Can you work these out from the model? Positions are in its coordinate system, mm. A direction names the side the tool comes from. Give positions to 0.01 mm unless a question says otherwise; leave off trailing zeros. Order: outer loops, then holes, each group sorted by start corner. A loop starts at its lowest first (then second) coordinate and runs counter-clockwise, first axis right, second up. Notation, with made-up numbers: (38.5, 64.25) - (84.5, 64.25) arc R18 ccw to (84.5, 90.25) - close; hole circle Ø2 at (0.5, 20). An arc over 180 degrees is marked (long way). Answer as CSV lines item,"result".
```python
from build123d import *

# Parameters (mm, degrees)
SKETCH1_W           = 24.825
SKETCH1_H           = 3.175
SKETCH1_W_2         = 3.175
SKETCH1_H_2         = 24.825
BOSS_EXTRUDE1_DEPTH = 60
SKETCH2_W           = 3.125
SKETCH2_H           = 5.4
BOSS_EXTRUDE4_DEPTH = 3.175
SKETCH4_R           = 8
CUT_EXTRUDE1_DEPTH  = 3.175
SKETCH3_R           = 8
CUT_EXTRUDE2_DEPTH  = 3.175
SKETCH5_W           = 3.175
SKETCH5_H           = 5.4
BOSS_EXTRUDE5_DEPTH = 3.175
SKETCH6_R           = 1.75
CUT_EXTRUDE3_DEPTH  = 10
SKETCH7_R           = 1.75
CUT_EXTRUDE4_DEPTH  = 10


with BuildPart() as part:
    # Sketch1 → Boss-Extrude1 (new body)
    with BuildSketch(Plane(origin=(0, 0, 0), x_dir=(1, 0, 0), z_dir=(0, 1, 0))):
        with Locations((-38.0875, 24.0875)):
            Rectangle(SKETCH1_W, SKETCH1_H)
        with Locations((-24.0875, 24.0875)):
            Rectangle(SKETCH1_W_2, SKETCH1_H)
        with Locations((-24.0875, 38.0875)):
            Rectangle(SKETCH1_W_2, SKETCH1_H_2)
    extrude(amount=BOSS_EXTRUDE1_DEPTH)

    # Sketch2 → Boss-Extrude4 (add)
    with BuildSketch(Plane.XY.offset(-22.5)):
        with Locations((-42.1875, -2.7)):
            Rectangle(SKETCH2_W, SKETCH2_H)
        with Locations((-31.5625, -2.7)):
            Rectangle(SKETCH2_W, SKETCH2_H)
    extrude(amount=-BOSS_EXTRUDE4_DEPTH)

    # Sketch4 → Cut-Extrude1 (cut)
    with BuildSketch(Plane.XY.offset(-22.5)):
        with Locations((-37.5, 30)):
            Circle(SKETCH4_R)
    extrude(amount=-CUT_EXTRUDE1_DEPTH, mode=Mode.SUBTRACT)

    # Sketch3 → Cut-Extrude2 (cut)
    with BuildSketch(Plane(origin=(-22.5, 0, 0), x_dir=(0, 0, -1), z_dir=(1, 0, 0))):
        with Locations((37.5, 30)):
            Circle(SKETCH3_R)
    extrude(amount=-CUT_EXTRUDE2_DEPTH, mode=Mode.SUBTRACT)

    # Sketch5 → Boss-Extrude5 (add)
    with BuildSketch(Plane(origin=(-22.5, 0, 0), x_dir=(0, 0, -1), z_dir=(1, 0, 0))):
        with Locations((42.2625, -2.7)):
            Rectangle(SKETCH5_W, SKETCH5_H)
        with Locations((31.5875, -2.7)):
            Rectangle(SKETCH5_W, SKETCH5_H)
    extrude(amount=-BOSS_EXTRUDE5_DEPTH)

    # Sketch6 → Cut-Extrude3 (cut)
    with BuildSketch(Plane.XY.offset(-22.5)):
        with Locations((-47.5, 45)):
            Circle(SKETCH6_R)
        with Locations((-27.5, 45)):
            Circle(SKETCH6_R)
    extrude(amount=-CUT_EXTRUDE3_DEPTH, mode=Mode.SUBTRACT)

    # Sketch7 → Cut-Extrude4 (cut)
    with BuildSketch(Plane(origin=(-22.5, 0, 0), x_dir=(0, 0, -1), z_dir=(1, 0, 0))):
        with Locations((47.5, 45)):
            Circle(SKETCH7_R)
        with Locations((27.5, 45)):
            Circle(SKETCH7_R)
    extrude(amount=-CUT_EXTRUDE4_DEPTH, mode=Mode.SUBTRACT)


solid = part.part
```
1) I'm going to push flat-ended pins straight in: P1, Ø4, axis at x = -28, z = -46, coming from the -Y side; P2, Ø3.5, axis at x = -24, y = -3, coming from the +Z side; P3, Ø12.5, axis at x = -41.5, y = 24, coming from the -Z side (3 decimals); P4, Ø3.5, axis at x = -24, z = -47.5, coming from the -Y side. Where does each tip first touch, or does it pass through?
Answer block:
P1,"through"
P2,"z = -30"
P3,"z = -25.675"
P4,"y = 0"
2) I want a section at C-C on y = 45. Write out the boundary of the cut face in (x, z) (3 decimals).
Answer block:
outline,"(-50.5, -25.675) - (-49.25, -25.675) - (-49.25, -22.5) - (-50.5, -22.5) - close; (-45.75, -25.675) - (-29.25, -25.675) - (-29.25, -22.5) - (-45.75, -22.5) - close; (-25.75, -25.675) - (-25.675, -25.675) - (-25.675, -25.75) - (-22.5, -25.75) - (-22.5, -22.5) - (-25.75, -22.5) - close; (-25.675, -50.5) - (-22.5, -50.5) - (-22.5, -49.25) - (-25.675, -49.25) - close; (-25.675, -45.75) - (-22.5, -45.75) - (-22.5, -29.25) - (-25.675, -29.25) - close"
3) I want a section at A-A on y = 30. Write out the boundary of the cut face in (x, z) (3 decimals), plus the area to 3 significant figures.
Answer block:
outline,"(-50.5, -25.675) - (-45.5, -25.675) - (-45.5, -22.5) - (-50.5, -22.5) - close; (-29.5, -25.675) - (-25.675, -25.675) - (-25.675, -29.5) - (-22.5, -29.5) - (-22.5, -22.5) - (-29.5, -22.5) - close; (-25.675, -50.5) - (-22.5, -50.5) - (-22.5, -45.5) - (-25.675, -45.5) - close"
area,"66.1 mm2"
4) Which directions (+Z, -Z, +X, -X, +Y, -Y) give clear straight access to the entire face, cutting with the end or side of a thin tool? Please do faces 5 (the flat face through (-24, 0, -47)), 6 (the flat face through (-24, -3, -30)), 7 (the flat face through (-33.125, -3, -24)), 8 (the flat face through (-47, 0, -24)), 9 (the flat face through (-25.675, 26.8, -29.6)).
Answer block:
face 5,"-Z, +X, -X, -Y"
face 6,"+Z, +X, -X, -Y"
face 7,"+Z, -Z, -Y"
face 8,"+Z, -Z, -X, -Y"
face 9,"-Z, -X, +Y, -Y"
5) I want a section at D-D on x = -48.25. Write out the boundary of the cut face in (y, z) (3 decimals).
Answer block:
outline,"(0, -25.675) - (43.419, -25.675) - (43.419, -22.5) - (0, -22.5) - close; (46.581, -25.675) - (60, -25.675) - (60, -22.5) - (46.581, -22.5) - close"
6) I need wall thicknesses on line 1 along Y through (x, z) = (-27.5, -23.2); line 2 along X through (y, z) = (8.5, -43.75) (3 decimals). Which ranges of each line are inside material? Lowest first, please. Write a range as [from, to].
Answer block:
line 1,"[0, 43.25], [46.75, 60]"
line 2,"[-25.675, -22.5]"
7) If we mould it in two halves opening along Z, with no side actions, what happens to faces 1 (the cylindrical face through (-24.07, 43.94, -26.11)), 2 (the flat face through (-30, -3, -24)), 3 (the flat face through (-24, 0, -37)), 4 (the flat face through (-30, 34, -22.5))? For each: +Z half, -Z half, draft (parallel to the pull), parting line (faces both ways), or undercut.
Answer block:
face 1,"undercut"
face 2,"draft"
face 3,"undercut"
face 4,"+Z half"
8) I want a section at B-B on z = -37.5. Write out the boundary of the cut face in (x, y) (3 decimals).
Answer block:
outline,"(-25.675, 0) - (-22.5, 0) - (-22.5, 22) - (-25.675, 22) - close; (-25.675, 38) - (-22.5, 38) - (-22.5, 60) - (-25.675, 60) - close"
